```python
from build123d import *

# Parameters (mm, degrees)
SKETCH1_W           = 90
SKETCH1_H           = 95
BOSS_EXTRUDE3_DEPTH = 15
SKETCH5_W           = 15
SKETCH5_H           = 8.4
CUT_EXTRUDE3_DEPTH  = 40
SKETCH7_W           = 95
SKETCH7_H           = 15
BOSS_EXTRUDE4_DEPTH = 5


with BuildPart() as part:
    # Sketch1 → Boss-Extrude3 (new body)
    with BuildSketch(Plane(origin=(0, 0, 0), x_dir=(1, 0, 0), z_dir=(0, 1, 0))):
        Rectangle(SKETCH1_W, SKETCH1_H)
    extrude(amount=BOSS_EXTRUDE3_DEPTH)

    # Sketch5 → Cut-Extrude3 (cut)
    with BuildSketch(Plane(origin=(45, 0, 0), x_dir=(0, 0, -1), z_dir=(1, 0, 0))):
        with Locations((0.9, 6.2)):
            Rectangle(SKETCH5_W, SKETCH5_H)
    extrude(amount=-CUT_EXTRUDE3_DEPTH, mode=Mode.SUBTRACT)

    # Sketch7 → Boss-Extrude4 (add)
    with BuildSketch(Plane(origin=(45, 0, 0), x_dir=(0, 0, -1), z_dir=(1, 0, 0))):
        with Locations((0, 7.5)):
            Rectangle(SKETCH7_W, SKETCH7_H)
    extrude(amount=BOSS_EXTRUDE4_DEPTH)


solid = part.part
```
The model under review builds one solid part; all positions refer to its coordinate system, in mm. A direction names the side the tool comes from. Coordinates: 2 decimals unless noted, no trailing zeros. Order: outer loops, then holes, each group sorted by start corner. A loop starts at its lowest first (then second) coordinate and runs counter-clockwise, first axis right, second up. Notation, with made-up numbers: (-30.5, 21) -> (-21.5, 21) arc R24 cw to (-21.5, 40) -> close; hole circle Ø9 at (36, 50). An arc over 180 degrees is marked (long way). Answer in a Markdown table with one row per item. Add a question column.
Item 1: Machinability: for faces 1 (the flat face through (-45, 7, 1)), 2 (the flat face through (25, 10.4, -1)), which of the approach directions +Z, -Z, +X, -X, +Y, -Y give a long, thin tool a straight path to every point of the face, cutting with its end or side? Answer none if there is none.
Item 2: We need section B-B on z = -2. Write out the cut boundary in (x, y), plus the area to 3 significant figures.
Item 3: To check wall thickness, follow probe 1 along Y at (x, z) = (42, 1); probe 2 along X at (y, z) = (9, -7.5); probe 3 along Z at (x, y) = (10, 5.75). State the ranges of each line that lie inside material, in increasing order.
Item 4: We need section A-A on x = 22.5. Write out the cut boundary in (y, z), plus the area to 3 significant figures.
Item 5: Mouldability with a two-part tool opening along Y and no side actions: class faces 3 (the flat face through (5, 6, -1)), 4 (the flat face through (2, 7, 47.5)), 5 (the flat face through (2, 0, 1)) as +Y half, -Y half, draft (parallel to the pull), parting line (faces both ways), or undercut.
Final values:
| question | item | result |
|---|---|---|
| 1 | face 1 | +Z, -Z, -X, +Y, -Y |
| 1 | face 2 | none |
| 2 | outline | (-45, 0) -> (50, 0) -> (50, 15) -> (-45, 15) -> close; hole (5, 2) -> (45, 2) -> (45, 10.4) -> (5, 10.4) -> close |
| 2 | area | 1,090 mm2 |
| 3 | probe 1 | y = 0 to 2, 10.4 to 15 |
| 3 | probe 2 | x = -45 to 5, 45 to 50 |
| 3 | probe 3 | z = -47.5 to -8.4, 6.6 to 47.5 |
| 4 | outline | (0, -47.5) -> (15, -47.5) -> (15, 47.5) -> (0, 47.5) -> close; hole (2, -8.4) -> (10.4, -8.4) -> (10.4, 6.6) -> (2, 6.6) -> close |
| 4 | area | 1,300 mm2 |
| 5 | face 3 | undercut |
| 5 | face 4 | draft |
| 5 | face 5 | -Y half |
